Input: part model. Units: mm. Frame: model coordinates. Face numbers are marked on the shaded views. A direction names the side the tool comes from. Round coordinates to 2 decimals unless told otherwise and drop trailing zeros. Loops run counter-clockwise (first coordinate to the right, second up) from the corner with the lowest first, then second, coordinate; pieces in that order, holes last. Notation, with made-up numbers: M 65.5,-18 L 124.5,-18 A5 cw 124.5,-10 Z; hole C -31,74 d10. An arc over 180 degrees is marked long. Return JSON: item names as keys, results as strings. Group by question number.
1) Section D-D (y = -40). Output: boundary loops of the cut face in (x, z) (3 decimals), plus the area to 3 significant figures.
2) Access query for the marked faces 1 and 2. Directions: +Z, -Z, +X, -X, +Y, -Y. A direction counts if a zero-diameter tool reaches every point of the face in a straight line with its end or side. Return the directions, or none.
3) Section C-C (y = -34.5). Output: boundary loops of the cut face in (x, z) (3 decimals).
4) Section A-A (x = 19.5). Count the separate pieces of the cut face and the enclosed holes in it, plus the area to 3 significant figures.
5) Material intervals for line 1 (Y direction, x = 13.25, z = 5.5); line 2 (Z direction, x = 18.5, y = -29); line 3 (Y direction, x = 20, z = 7.25), sorted ascending. Write a range as from..to.
6) Mould query, pull axis Z, two halves, no side actions, for the marked faces 3, 4 and 5. Classes: +Z half, -Z half, draft (parallel to the pull), parting line (faces both ways), or undercut.
7) Contact query for flat-ended pins moving along their axis: P1, Ø4.5, axis at y = -4.76, z = 4.76, coming from the -X side; P2, Ø1, axis at x = 5, z = 2.5, coming from the +Y side. Output: stop coordinate, or through.
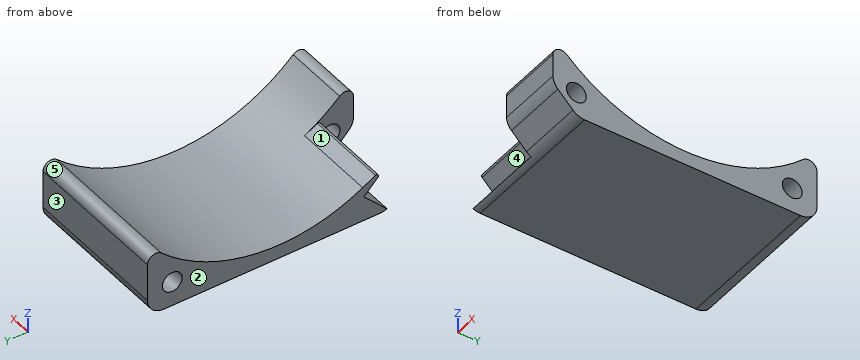
from build123d import *

# Parameters (mm, degrees)
BOSS_EXTRUDE1_DEPTH = 28.575
CHAMFER1_SIZE       = 4.7625
FILLET3_R           = 3.175
CUT_EXTRUDE1_START  = -12.7
CUT_EXTRUDE1_DEPTH  = 48.337684469
FILLET4_R           = 0.396875
FILLET5_R           = 3.175
FILLET6_R           = 1.5875
SKETCH3_R           = 1.905
CUT_EXTRUDE2_DEPTH  = 60.514034165


with BuildPart() as part:
    # Sketch1 → Boss-Extrude1 (new body)
    with BuildSketch(Plane(origin=(0, 0, 0), x_dir=(0, 0, -1), z_dir=(1, 0, 0))):
        with BuildLine():
            Line((0, 0), (-14.399754562, 0))
            ThreePointArc((-14.399754562, 0), (-2.654588994, -25.4), (-14.399754562, -50.8))
            Line((-14.399754562, -50.8), (0, -50.8))
            Line((0, -50.8), (0, 0))
        make_face()
    extrude(amount=BOSS_EXTRUDE1_DEPTH)

    # Chamfer1
    chamfer1_edges = [part.edges().sort_by_distance(p)[0] for p in [
        (14.2875, -50.8, 0),
    ]]
    chamfer(chamfer1_edges, length=CHAMFER1_SIZE)

    # Fillet3
    fillet3_edges = [part.edges().sort_by_distance(p)[0] for p in [
        (14.2875, -46.0375, 0),
        (14.2875, -50.8, 4.7625),
    ]]
    fillet(fillet3_edges, radius=FILLET3_R)

    # Sketch2 → Cut-Extrude1 (cut, through all)
    with BuildSketch(Plane(origin=(28.575, 0, 0), x_dir=(0, 0, -1), z_dir=(1, 0, 0)).offset(CUT_EXTRUDE1_START)):
        with BuildLine():
            Line((-9.432233183, -46.30987194), (-6.747973263, -41.405330404))
            ThreePointArc((-6.747973263, -41.405330404), (-10.143469679, -46.453213193), (-14.399754562, -50.8))
            Line((-14.399754562, -50.8), (-6.077628061, -50.8))
            ThreePointArc((-6.077628061, -50.8), (-4.862608163, -50.558317516), (-3.83256403, -49.87006403))
            Line((-3.83256403, -49.87006403), (-0.92993597, -46.96743597))
            ThreePointArc((-0.92993597, -46.96743597), (-0.583051244, -46.556064021), (-0.31061766, -46.092021096))
            Line((-0.31061766, -46.092021096), (-4.7625, -41.640138757))
            Line((-4.7625, -41.640138757), (-9.432233183, -46.30987194))
        make_face()
    extrude(amount=-CUT_EXTRUDE1_DEPTH, mode=Mode.SUBTRACT)

    # Fillet4
    fillet4_edges = [part.edges().sort_by_distance(p)[0] for p in [
        (7.9375, -46.30987194, 9.432233183),
    ]]
    fillet(fillet4_edges, radius=FILLET4_R)

    # Fillet5
    fillet5_edges = [part.edges().sort_by_distance(p)[0] for p in [
        (14.2875, 0, 0),
    ]]
    fillet(fillet5_edges, radius=FILLET5_R)

    # Fillet6
    fillet6_edges = [part.edges().sort_by_distance(p)[0] for p in [
        (22.225, -50.8, 14.399754562),
        (14.2875, 0, 14.399754562),
    ]]
    fillet(fillet6_edges, radius=FILLET6_R)

    # Sketch3 → Cut-Extrude2 (cut, through all)
    with BuildSketch(Plane(origin=(28.575, 0, 0), x_dir=(0, 0, -1), z_dir=(1, 0, 0))):
        with Locations((-4.7625, -4.7625)):
            Circle(SKETCH3_R)
        with Locations((-4.7625, -46.309871939)):
            Circle(SKETCH3_R)
    extrude(amount=-CUT_EXTRUDE2_DEPTH, mode=Mode.SUBTRACT)


solid = part.part
Returned:
{
 "1": {"outline": "M 0,0 L 28.575,0 L 28.575,6.022 L 0,6.022 Z", "area": "172 mm^2"},
 "2": {"face 1": "+Z, -X", "face 2": "+Z, -Z, -X, +Y, -Y"},
 "3": {"outline": "M 0,0 L 28.575,0 L 28.575,3.921 L 0,3.921 Z"},
 "4": {"separate pieces": "1", "enclosed holes": "2", "area": "274 mm^2"},
 "5": {"line 1": "y = -42.38..-38.88, -11.92..-6.52, -3.01..0", "line 2": "z = 0..2.85", "line 3": "y = -50.8..-42.29, -8.51..0"},
 "6": {"face 3": "draft", "face 4": "undercut", "face 5": "+Z half"},
 "7": {"P1": "stops at x = 0", "P2": "stops at y = 0"}
}
